Autodesk Inventor part; units mm, degrees
ref_plane "YZ Plane" through (0, 0, 0) normal (1, 0, 0) x (0, 1, 0)
ref_plane "XZ Plane" through (0, 0, 0) normal (0, 1, 0) x (-1, 0, 0)
ref_plane "XY Plane" through (0, 0, 0) normal (0, 0, 1) x (1, 0, 0)
sketch "Sketch1" plane through (0, 0, 0) normal (0, 0, 1) x (1, 0, 0)
  line L0 (-37.5, -42.6) -> (37.5, -42.6)
  line L1 (37.5, -42.6) -> (37.5, 42.6)
  line L2 (37.5, 42.6) -> (-37.5, 42.6)
  line L3 (-37.5, 42.6) -> (-37.5, -42.6)
  line L4 (-37.5, -42.6) -> (37.5, 42.6) construction
  line L5 (37.5, -42.6) -> (-37.5, 42.6) construction
  point P0 (0, 0)
  dimension "d0" = 75
  dimension "d1" = 85.2
extrude "Extrusion1" add sketch "Sketch1" along normal blind 10
sketch "Sketch4" plane through (0, 0, 10) normal (0, 0, 1) x (1, 0, 0)
  point P0 (0, 0)
sketch "Sketch5" plane through (0, 0, 10) normal (0, 0, 1) x (1, 0, 0)
  line L0 (-37.5, -42.6) -> (37.5, -42.6)
  line L1 (0, -42.6) -> (0, 1.6)
  circle A0 centre (0, 1.6) radius 7.5
  line L2 (0, 1.6) -> (13, 1.6)
  point P0 (0, 0)
  dimension "d21" = 44.2
  dimension "d22" = 15
extrude "Extrusion6" cut sketch "Sketch5" against normal blind 10
sketch "Sketch6" plane through (0, 0, 10) normal (0, 0, 1) x (1, 0, 0)
  circle A0 centre (13, 6.6) radius 3.75
sketch "Boceto8" plane through (0, 0, 10) normal (0, 0, 1) x (1, 0, 0)
  circle A0 centre (-9.5, 7.6) radius 2.5
sketch "Boceto9" plane through (0, 0, 0) normal (0, 0, -1) x (-1, 0, 0)
  circle A0 centre (9.5, 7.6) radius 2.5
sketch "Boceto10" plane through (0, 0, 10) normal (0, 0, 1) x (1, 0, 0)
  circle A0 centre (-9.5, 7.6) radius 2.5
sketch "Boceto11" plane through (0, 0, 0) normal (0, 0, -1) x (-1, 0, 0)
  circle A0 centre (9.5, 7.6) radius 2.5
sketch "Sketch12" plane through (0, 0, 10) normal (0, 0, 1) x (1, 0, 0)
  point P0 (0, 0)
sketch "Sketch15" plane through (0, 0, 0) normal (0, 0, -1) x (-1, 0, 0)
  circle A0 centre (32.5, 37.6) radius 2
  circle A1 centre (32.5, 37.6) radius 3.61
  line L0 (-37.5, 42.6) -> (37.5, 42.6)
  line L1 (0, 42.6) -> (0, 0)
  line L2 (-37.5, -42.6) -> (-37.5, 42.6)
  line L3 (-37.5, 0) -> (37.5, 0)
  circle A2 centre (-32.5, 37.6) radius 2
  circle A3 centre (-32.5, 37.6) radius 3.61
  circle A4 centre (32.5, -37.6) radius 2
  circle A5 centre (32.5, -37.6) radius 3.61
  circle A6 centre (-32.5, -37.6) radius 2
  circle A7 centre (-32.5, -37.6) radius 3.61
  point P0 (0, -42.6)
  dimension "d52" = 7.22
extrude "Extrusion10" cut sketch "Sketch15" against normal blind 4.5 contours A0 | A1 | A3 | A4 | A5 | A6 | A7
sketch "Sketch13" plane through (0, 0, 10) normal (0, 0, 1) x (1, 0, 0)
  line L0 (37.5, -42.6) -> (37.5, 42.6)
  line L1 (37.5, -42.6) -> (32.5, -42.6)
  line L2 (-37.5, -42.6) -> (37.5, -42.6)
  line L3 (32.5, -42.6) -> (32.5, -37.6)
  circle A0 centre (32.5, -37.6) radius 2.15
  circle A1 centre (32.5, -37.6) radius 3.61
  line L4 (0, 0) -> (0, -42.6)
  line L5 (-37.5, 42.6) -> (-37.5, -42.6)
  line L6 (-37.5, 0) -> (37.5, 0)
  line L7 (-32.5, -42.6) -> (-32.5, -37.6)
  circle A2 centre (-32.5, -37.6) radius 2.15
  circle A3 centre (-32.5, -37.6) radius 3.61
  line L8 (37.5, 42.6) -> (32.5, 42.6)
  line L9 (-37.5, 42.6) -> (37.5, 42.6)
  line L10 (32.5, 42.6) -> (32.5, 37.6)
  circle A4 centre (32.5, 37.6) radius 2.15
  circle A5 centre (32.5, 37.6) radius 3.61
  line L11 (-32.5, 42.6) -> (-32.5, 37.6)
  circle A6 centre (-32.5, 37.6) radius 2.15
  circle A7 centre (-32.5, 37.6) radius 3.61
  line L12 (32.5, -37.6) -> (32.5, -27.6)
  circle A8 centre (32.5, -27.6) radius 2.15
  circle A9 centre (32.5, -27.6) radius 3.61
  line L13 (-37.5, -42.6) -> (-37.5, 42.6)
  line L14 (-37.5, -42.6) -> (-32.5, -42.6)
  line L15 (37.5, -42.6) -> (-37.5, -42.6)
  line L16 (-32.5, -42.6) -> (-32.5, -37.6)
  circle A10 centre (-32.5, -37.6) radius 2.15
  circle A11 centre (-32.5, -37.6) radius 3.61
  line L17 (-32.5, -37.6) -> (-32.5, -27.6)
  circle A12 centre (-32.5, -27.6) radius 2.15
  circle A13 centre (-32.5, -27.6) radius 3.61
  circle A14 centre (32.5, 27.6) radius 2.15
  circle A15 centre (32.5, 27.6) radius 3.61
  circle A16 centre (-32.5, 27.6) radius 2.15
  circle A17 centre (-32.5, 27.6) radius 3.61
  point P0 (0, 42.6)
  dimension "d43" = 5
  dimension "d44" = 5
  dimension "d45" = 4.3
  dimension "d46" = 7.22
  dimension "d55" = 10
  dimension "d56" = 4.3
  dimension "d57" = 7.22
extrude "Extrusion11" cut sketch "Sketch13" against normal blind 10 contours A8 | A4 | A6 | A12 | A0 L12 L3 | L3 L12 A0 | A2 L17 L7 | L7 L17 A2 | A14 | A16
sketch "Sketch16" plane through (0, 0, 0) normal (0, 0, -1) x (-1, 0, 0)
  circle A0 centre (-32.5, 27.6) radius 2.15
  circle A1 centre (-32.5, 27.6) radius 3.61
  circle A2 centre (32.5, 27.6) radius 2.15
  circle A3 centre (32.5, 27.6) radius 3.61
  circle A4 centre (-32.5, -27.6) radius 2.15
  circle A5 centre (-32.5, -27.6) radius 3.61
  circle A6 centre (32.5, -27.6) radius 2.15
  circle A7 centre (32.5, -27.6) radius 3.61
  point P0 (0, 0)
  dimension "d60" = 7.22
  dimension "d61" = 7.22
  dimension "d62" = 7.22
  dimension "d63" = 7.22
extrude "Extrusion12" cut sketch "Sketch16" against normal blind 4.5
properties part number "Rb PEEK - Corto con ventana"
Work out the finished part from the listing and answer in its coordinate system (mm). A direction names the side the tool comes from. Round coordinates to 2 decimals unless told otherwise and drop trailing zeros. Loops run counter-clockwise (first coordinate to the right, second up) from the corner with the lowest first, then second, coordinate; pieces in that order, holes last. Notation, with made-up numbers: (-16, 15) - (9, 15) arc R18 cw to (9, 21) - close; hole circle Ø11 at (21, 88.5). An arc over 180 degrees is marked (long way). One line per item, written item: value.
Q1. Find section B-B on x = 0. Give the vertices of the cut face in (y, z), and give its area (3 significant figures).
Check values:
outline: (-42.6, 0) - (-5.9, 0) - (-5.9, 10) - (-42.6, 10) - close; (9.1, 0) - (42.6, 0) - (42.6, 10) - (9.1, 10) - close
area: 702 mm2
Q2. For faces 3 (the flat face through (33, 25, 4.5)), 4 (the cylindrical face through (-30.514, -28.423, 7.288)), determine the directions among +Z, -Z, +X, -X, +Y, -Y from which every point of the face is accessible in a straight line to the end or side of a thin tool.
Check values:
face 3: -Z
face 4: +Z, -Z
Q3. The mould has two halves that part along X. Classify faces 1 (the flat face through (8, 1, 0)), 2 (the flat face through (-32, -30, 4.5)): +X half, -X half, draft (parallel to the pull), parting line (faces both ways), or undercut.
Check values:
face 1: draft
face 2: undercut
Q4. Each of these flat-tipped pins is pushed along its axis until it touches: pin 1 Ø4.5 at (x, y) = (-32.5, 27.6) entering from -Z; pin 2 Ø2.5 at (x, y) = (32.5, -27.6) entering from +Z. Where does it stop, or does it pass through?
Check values:
pin 1: z = 4.5
pin 2: through
Q5. Find section C-C on y = 27.6. Give the vertices of the cut face in (x, z).
Check values:
outline: (-37.5, 0) - (-36.11, 0) - (-36.11, 4.5) - (-34.65, 4.5) - (-34.65, 10) - (-37.5, 10) - close; (-30.35, 4.5) - (-28.89, 4.5) - (-28.89, 0) - (28.89, 0) - (28.89, 4.5) - (30.35, 4.5) - (30.35, 10) - (-30.35, 10) - close; (34.65, 4.5) - (36.11, 4.5) - (36.11, 0) - (37.5, 0) - (37.5, 10) - (34.65, 10) - close
Q6. Straight lines are drawn through the part: probe 1 along Y at (x, z) = (-32.5, 6.2); probe 2 along X at (y, z) = (-37.5, 5); probe 3 along Y at (x, z) = (-32.5, 2.15). For each, find the intervals that lie inside material, in ascending order.
Check values:
probe 1: -42.6 to -39.75, -35.45 to -29.75, -25.45 to 25.45, 29.75 to 35.45, 39.75 to 42.6
probe 2: -37.5 to -34.65, -30.35 to 30.35, 34.65 to 37.5
probe 3: -42.6 to -41.21, -33.99 to -31.21, -23.99 to 23.99, 31.21 to 33.99, 41.21 to 42.6
Q7. Find section A-A on z = 2. State how many separate pieces and enclosed holes the cut face has, and give its area (3 significant figures).
Check values:
separate pieces: 1
enclosed holes: 9
area: 5,890 mm2
